Check sheet for the modelled part. Datum: model origin and axes. Units: mm. A direction names the side the tool comes from. Round coordinates to 2 decimals unless told otherwise and drop trailing zeros. Loops run counter-clockwise (first coordinate to the right, second up) from the corner with the lowest first, then second, coordinate; pieces in that order, holes last. Notation, with made-up numbers: (86, 4) - (138, 4) arc R34 cw to (138, 37) - close; hole circle Ø2 at (15.25, 57.25). An arc over 180 degrees is marked (long way). Put each result on its own line as item: value.
```python
from build123d import *

# Parameters (mm, degrees)
SKETCH1_R           = 75
BOSS_EXTRUDE1_DEPTH = 50
SHELL1_T            = 1.6
SKETCH2_R           = 21
CUT_EXTRUDE1_DEPTH  = 50
SKETCH3_R           = 1.75
CUT_EXTRUDE2_DEPTH  = 50
SKETCH4_R           = 3
CUT_EXTRUDE3_DEPTH  = 50


with BuildPart() as part:
    # Sketch1 → Boss-Extrude1 (new body)
    with BuildSketch(Plane(origin=(0, 0, 0), x_dir=(1, 0, 0), z_dir=(0, 1, 0))):
        with Locations(Location((0, 0, 0), (0, 0, 270))):
            Circle(SKETCH1_R)
    extrude(amount=BOSS_EXTRUDE1_DEPTH)

    # Shell1
    shell1_openings = [part.faces().sort_by_distance(p)[0] for p in [
        (0, 50, 0),
    ]]
    offset(amount=SHELL1_T, openings=shell1_openings, kind=Kind.INTERSECTION)

    # Sketch2 → Cut-Extrude1 (cut)
    with BuildSketch(Plane(origin=(0, 0, 0), x_dir=(1, 0, 0), z_dir=(0, 1, 0))):
        with Locations(Location((0, 54, 0), (0, 0, 270))):
            Circle(SKETCH2_R)
    extrude(amount=-CUT_EXTRUDE1_DEPTH, mode=Mode.SUBTRACT)

    # Sketch3 → Cut-Extrude2 (cut)
    with BuildSketch(Plane(origin=(0, 0, 0), x_dir=(1, 0, 0), z_dir=(0, 1, 0))):
        with Locations(Location((0, 28, 0), (0, 0, 270))):
            Circle(SKETCH3_R)
        with Locations(Location((-22.516660498, 67, 0), (0, 0, 270))):
            Circle(SKETCH3_R)
        with Locations(Location((22.516660498, 67, 0), (0, 0, 270))):
            Circle(SKETCH3_R)
    extrude(amount=-CUT_EXTRUDE2_DEPTH, mode=Mode.SUBTRACT)

    # Sketch4 → Cut-Extrude3 (cut)
    with BuildSketch(Plane(origin=(0, 0, 0), x_dir=(1, 0, 0), z_dir=(0, 1, 0))):
        with Locations(Location((0, 0, 0), (0, 0, 270))):
            Circle(SKETCH4_R)
    extrude(amount=-CUT_EXTRUDE3_DEPTH, mode=Mode.SUBTRACT)


solid = part.part
```
Item 1: Go/stop test with flat-tipped pins: pin 1 (8 mm diameter, centred on y = 17.5, z = 35.5, fed in from -X); pin 2 (12 mm diameter, centred on x = -54, y = 22.5, fed in from +Z); pin 3 (8 mm diameter, centred on y = 13, z = -44, fed in from +X). Record where each tip stops, or that it passes through.
Filled sheet:
pin 1: x = -69.82
pin 2: z = 59.7
pin 3: x = 65.33
Item 2: Thickness scan on line 1 (X direction, y = -0.6, z = -67); line 2 (Y direction, x = -30.5, z = -25.5); line 3 (X direction, y = 8.5, z = -8). Record the ranges inside material, lowest first. Write a range as from..to.
Filled sheet:
line 1: -37.13..-24.27, -20.77..-16.49, 16.49..20.77, 24.27..37.13
line 2: -1.6..0
line 3: -76.18..-74.57, 74.57..76.18
Item 3: Section check B-B on x = -6. Enter the section's corners in (y, z), then the cut area to 3 significant figures.
Filled sheet:
outline: (-1.6, -76.36) - (50, -76.36) - (50, -74.76) - (0, -74.76) - (0, -74.12) - (-1.6, -74.12) - close; (-1.6, -33.88) - (0, -33.88) - (0, 74.76) - (50, 74.76) - (50, 76.36) - (-1.6, 76.36) - close
area: 340 mm²
Item 4: Tool access check on faces 4 (the flat face through (1, 0, 16)), 5 (the cylindrical face through (0.92, -0.79, -74.98)). Record the directions out of +Z, -Z, +X, -X, +Y, -Y that give a thin tool (end or side, any length) a straight path to the whole face; none if there is none.
Filled sheet:
face 4: +Y
face 5: +Y, -Y
Item 5: Section check A-A on z = 0. Enter the section's corners in (x, y), then the cut area to 3 significant figures.
Filled sheet:
outline: (-76.6, -1.6) - (-3, -1.6) - (-3, 0) - (-75, 0) - (-75, 50) - (-76.6, 50) - close; (3, -1.6) - (76.6, -1.6) - (76.6, 50) - (75, 50) - (75, 0) - (3, 0) - close
area: 396 mm²
Item 6: Section check C-C on y = 37.5. Enter the section's corners in (x, z).
Filled sheet:
outline: circle Ø153.2 at (0, 0); hole circle Ø150 at (0, 0)
Item 7: Release check for a two-part mould opening along Z. For faces 1 (the flat face through (-56, 50, 51)), 2 (the cylindrical face through (23.009, 23.839, 73.063)), 3 (the cylindrical face through (0.08, -0.79, -29.75)) record: +Z half, -Z half, draft (parallel to the pull), parting line (faces both ways), or undercut.
Filled sheet:
face 1: draft
face 2: parting line
face 3: undercut
Item 8: Section check D-D on z = 45. Enter the section's corners in (x, y).
Filled sheet:
outline: (-61.99, -1.6) - (61.99, -1.6) - (61.99, 50) - (60, 50) - (60, 0) - (-60, 0) - (-60, 50) - (-61.99, 50) - close
